Can you work these out from the model? Positions are in its coordinate system, mm. A direction names the side the tool comes from. Round coordinates to 2 decimals unless told otherwise and drop trailing zeros. Write each loop counter-clockwise with the first axis right and the second up, starting at its lowest first coordinate (ties: lowest second). Pieces come first, ordered by that corner, then holes. Notation, with made-up numbers: M 35.5,-9 L 43.5,-9 A26 cw 43.5,19 Z; hole C 83,-11 d7. An arc over 180 degrees is marked long. Answer in a Markdown table with one row per item. Add a question column.
(1) If I drill on probe 1 along Y at (x, z) = (44, 5.3); probe 2 along Y at (x, z) = (44, 1.75); probe 3 along X at (y, z) = (-40, 3.75), over which ranges is the centre line in solid material (lowest first)?
(2) For faces 4 (the face through (-49.1, -1, 3)), 5 (the face through (-1, 1, 1.8)), 6 (the face through (46, -24, 3)), which set-ups out of +Z, -Z, +X, -X, +Y, -Y let a thin tool reach every point of the face, with its end or its side?
(3) Suppose I cut it at C-C, the plane y = -24. Count the separate pieces of the cut face and the enclosed holes in it, then the cut area to 3 significant figures.
(4) Suppose I cut it at A-A, the plane z = 6.75. Write out the boundary of the cut face in (x, y), then the cut area to 3 significant figures.
(5) Suppose I cut it at D-D, the plane x = 20. Write out the boundary of the cut face in (y, z), then the cut area to 3 significant figures.
(6) If we mould it in two halves opening along Y, with no side actions, what happens to faces 1 (the face through (49.1, -1, 3)), 2 (the face through (-1, 46.1, 3)), 3 (the face through (-44, 39.5, 3))? For each: released by +Y, released by -Y, zero draft, split by the parting line, or undercut.
(7) Suppose I cut it at B-B, the plane x = -11. Write out the boundary of the cut face in (y, z).
(8) I'm going to push flat-ended pins straight in: pin 1 (5.5 mm diameter, centred on x = -44, y = -24, fed in from -Z); pin 2 (1 mm diameter, centred on y = 35, z = 1, fed in from -X) (3 decimals); pin 3 (3 mm diameter, centred on x = 25, y = -26.5, fed in from +Z). Where does each tip first touch, or does it pass through?
from build123d import *

# Parameters (mm, degrees)
SKETCH007_W   = 98.2
SKETCH007_H   = 92.2
SKETCH007_R   = 3
SKETCH007_R_2 = 1.75
SKETCH007_W_2 = 21.5
SKETCH007_H_2 = 9.5
PAD006_DEPTH  = 1.8
SKETCH005_W   = 98.2
SKETCH005_H   = 92.2
SKETCH005_W_2 = 95
SKETCH005_H_2 = 89
PAD007_DEPTH  = 3
SKETCH008_R   = 4.5
SKETCH008_R_2 = 3
PAD008_DEPTH  = 1.2
SKETCH009_R   = 4.5
SKETCH009_R_2 = 1.75
PAD009_DEPTH  = 1.8
SKETCH006_R   = 2.9
SKETCH006_R_2 = 1.75
PAD010_DEPTH  = 3.2
FILLET002_R   = 1.799


with BuildPart() as part:
    # Sketch007 → Pad006 (new body)
    with BuildSketch(Plane.XY):
        Rectangle(SKETCH007_W, SKETCH007_H)
        with Locations((-44, 41.5)):
            Circle(SKETCH007_R, mode=Mode.SUBTRACT)
        with Locations((44, 41.5)):
            Circle(SKETCH007_R, mode=Mode.SUBTRACT)
        with Locations((44, -24)):
            Circle(SKETCH007_R, mode=Mode.SUBTRACT)
        with Locations((-44, -24)):
            Circle(SKETCH007_R, mode=Mode.SUBTRACT)
        with Locations((-20, -16.5)):
            Circle(SKETCH007_R_2, mode=Mode.SUBTRACT)
        with Locations((20, -16.5)):
            Circle(SKETCH007_R_2, mode=Mode.SUBTRACT)
        with Locations((15.5, 32.75)):
            Rectangle(SKETCH007_W_2, SKETCH007_H_2, mode=Mode.SUBTRACT)
        with Locations((-15.5, 32.75)):
            Rectangle(SKETCH007_W_2, SKETCH007_H_2, mode=Mode.SUBTRACT)
    extrude(amount=PAD006_DEPTH)

    # Sketch005 → Pad007 (new body)
    with BuildSketch(Plane.XY.offset(1.8)):
        Rectangle(SKETCH005_W, SKETCH005_H)
        Rectangle(SKETCH005_W_2, SKETCH005_H_2, mode=Mode.SUBTRACT)
    extrude(amount=PAD007_DEPTH)

    # Sketch008 → Pad008 (new body)
    with BuildSketch(Plane.XY.offset(1.8)):
        with Locations((-44, 41.5)):
            Circle(SKETCH008_R)
        with Locations((-44, 41.5)):
            Circle(SKETCH008_R_2, mode=Mode.SUBTRACT)
        with Locations((44, 41.5)):
            Circle(SKETCH008_R)
        with Locations((44, 41.5)):
            Circle(SKETCH008_R_2, mode=Mode.SUBTRACT)
        with Locations((44, -24)):
            Circle(SKETCH008_R)
        with Locations((44, -24)):
            Circle(SKETCH008_R_2, mode=Mode.SUBTRACT)
        with Locations((-44, -24)):
            Circle(SKETCH008_R)
        with Locations((-44, -24)):
            Circle(SKETCH008_R_2, mode=Mode.SUBTRACT)
    extrude(amount=PAD008_DEPTH)

    # Sketch009 → Pad009 (new body)
    with BuildSketch(Plane.XY.offset(3)):
        with Locations((-44, 41.5)):
            Circle(SKETCH009_R)
        with Locations((-44, 41.5)):
            Circle(SKETCH009_R_2, mode=Mode.SUBTRACT)
        with Locations((44, 41.5)):
            Circle(SKETCH009_R)
        with Locations((44, 41.5)):
            Circle(SKETCH009_R_2, mode=Mode.SUBTRACT)
        with Locations((44, -24)):
            Circle(SKETCH009_R)
        with Locations((44, -24)):
            Circle(SKETCH009_R_2, mode=Mode.SUBTRACT)
        with Locations((-44, -24)):
            Circle(SKETCH009_R)
        with Locations((-44, -24)):
            Circle(SKETCH009_R_2, mode=Mode.SUBTRACT)
    extrude(amount=PAD009_DEPTH)

    # Sketch006 → Pad010 (new body)
    with BuildSketch(Plane.XY.offset(4.8)):
        with Locations((-44, 41.5)):
            Circle(SKETCH006_R)
        with Locations((-44, 41.5)):
            Circle(SKETCH006_R_2, mode=Mode.SUBTRACT)
        with Locations((44, 41.5)):
            Circle(SKETCH006_R)
        with Locations((44, 41.5)):
            Circle(SKETCH006_R_2, mode=Mode.SUBTRACT)
        with Locations((44, -24)):
            Circle(SKETCH006_R)
        with Locations((44, -24)):
            Circle(SKETCH006_R_2, mode=Mode.SUBTRACT)
        with Locations((-44, -24)):
            Circle(SKETCH006_R)
        with Locations((-44, -24)):
            Circle(SKETCH006_R_2, mode=Mode.SUBTRACT)
    extrude(amount=PAD010_DEPTH)

    # Fillet002
    fillet002_edges = [part.edges().sort_by_distance(p)[0] for p in [
        (49.1, 0, 0),
        (0, -46.1, 0),
        (-49.1, 0, 0),
        (0, 46.1, 0),
        (-49.1, 46.1, 0.9),
        (-49.1, 46.1, 3.3),
        (-49.1, -46.1, 3.3),
        (-49.1, -46.1, 0.9),
        (49.1, -46.1, 3.3),
        (49.1, -46.1, 0.9),
        (49.1, 46.1, 0.9),
        (49.1, 46.1, 3.3),
    ]]
    fillet(fillet002_edges, radius=FILLET002_R)


solid = part.part
Calculated:
| question | item | result |
|---|---|---|
| 1 | probe 1 | -26.9 to -25.75, -22.25 to -21.1, 38.6 to 39.75, 43.25 to 44.4 |
| 1 | probe 2 | -46.1 to -27, -21 to 38.5, 44.5 to 46.1 |
| 1 | probe 3 | -49.1 to -47.5, 47.5 to 49.1 |
| 2 | face 4 | +Z, -Z, -X, +Y, -Y |
| 2 | face 5 | +Z |
| 2 | face 6 | -Z |
| 3 | separate pieces | 3 |
| 3 | enclosed holes | 0 |
| 3 | area | 199 mm² |
| 4 | outline | C -44,-24 d5.8; C -44,41.5 d5.8; C 44,-24 d5.8; C 44,41.5 d5.8; hole C -44,-24 d3.5; hole C -44,41.5 d3.5; hole C 44,-24 d3.5; hole C 44,41.5 d3.5 |
| 4 | area | 67.2 mm² |
| 5 | outline | M -46.1,1.8 A1.8 ccw -44.3,0 L -18.25,0 L -18.25,1.8 L -44.5,1.8 L -44.5,4.8 L -46.1,4.8 Z; M -14.75,0 L 28,0 L 28,1.8 L -14.75,1.8 Z; M 37.5,0 L 44.3,0 A1.8 ccw 46.1,1.8 L 46.1,4.8 L 44.5,4.8 L 44.5,1.8 L 37.5,1.8 Z |
| 5 | area | 151 mm² |
| 6 | face 1 | zero draft |
| 6 | face 2 | released by +Y |
| 6 | face 3 | undercut |
| 7 | outline | M -46.1,1.8 A1.8 ccw -44.3,0 L 28,0 L 28,1.8 L -44.5,1.8 L -44.5,4.8 L -46.1,4.8 Z; M 37.5,0 L 44.3,0 A1.8 ccw 46.1,1.8 L 46.1,4.8 L 44.5,4.8 L 44.5,1.8 L 37.5,1.8 Z |
| 8 | pin 1 | z = 3 |
| 8 | pin 2 | x = -49.075 |
| 8 | pin 3 | z = 1.8 |
